Here's how the part is built. I have some questions about the finished solid (model axes, mm). Face numbers are marked on the shaded views. A direction names the side the tool comes from. Round coordinates to 2 decimals unless told otherwise and drop trailing zeros. Loops run counter-clockwise (first coordinate to the right, second up) from the corner with the lowest first, then second, coordinate; pieces in that order, holes last. Notation, with made-up numbers: M 23,18 L 46,18 A17 cw 46,51 Z; hole C -1.75,43.25 d4. An arc over 180 degrees is marked long. Answer as CSV lines item,"result".
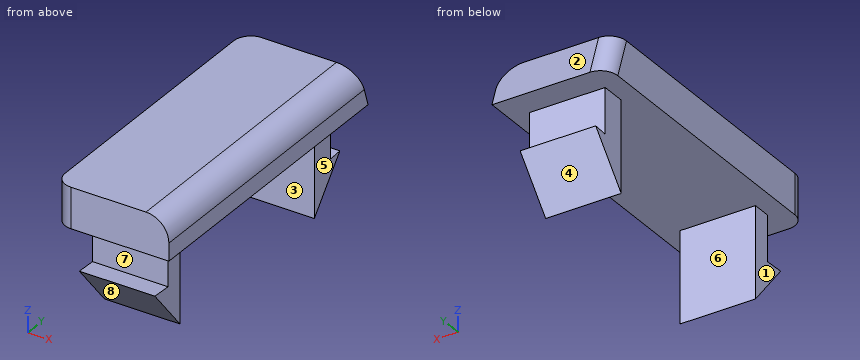
```python
from build123d import *

# Parameters (mm, degrees)
F1_DEPTH = 12.7
F2_DEPTH = 8.382
F3_R     = 3.679261
F4_R     = 5.08


with BuildPart() as f1:
    # F0 (on Right) → F1 (new body, symmetric)
    with BuildSketch(Plane.YZ):
        Polygon((30.308623, 31.392861), (-34.372479, 31.392861), (-34.724846, 31.392861), (-34.724846, 22.405792), (-28.332443, 22.405792), (-24.258062, 22.405792), (-20.550046, 22.405792), (-9.070974, 22.405792), (1.610943, 22.405792), (21.591455, 22.405792), (27.077377, 22.405792), (33.283076, 22.405792), align=None)
    extrude(amount=F1_DEPTH, both=True)

    # F0 (on Right) → F2 (join, symmetric)
    with BuildSketch(Plane.YZ):
        Polygon((30.308623, 31.392861), (-34.372479, 31.392861), (-34.724846, 31.392861), (-34.724846, 22.405792), (-28.332443, 22.405792), (-24.258062, 22.405792), (-20.550046, 22.405792), (-9.070974, 22.405792), (1.610943, 22.405792), (21.591455, 22.405792), (27.077377, 22.405792), (33.283076, 22.405792), align=None)
        Polygon((27.077377, 12.309055), (27.077377, 22.405792), (21.591455, 22.405792), (21.591455, 2.212318), (30.308623, 12.499893), align=None)
        Polygon((-24.258062, 22.405792), (-28.332443, 22.405792), (-28.332443, 12.309055), (-32.845773, 12.499893), (-24.258062, 2.212318), align=None)
    extrude(amount=F2_DEPTH, both=True)

    # F3
    f3_edges = [f1.edges().sort_by_distance(p)[0] for p in [
        (-12.7, -34.724846, 26.899327),
        (-12.7, 31.795849, 26.899327),
    ]]
    fillet(f3_edges, radius=F3_R)

    # F4
    f4_edges = [f1.edges().sort_by_distance(p)[0] for p in [
        (12.7, -2.208112, 31.392861),
    ]]
    fillet(f4_edges, radius=F4_R)


solid = f1.part
```
1. For P1, Ø8, axis at x = 0.5, z = 18, coming from the +Y side; P2, Ø2.5, axis at y = 24.5, z = 8, coming from the +X side; P3, Ø1, axis at x = -2, z = 20.5, coming from the -Y side, each with a flat end and sliding along its axis, tell me the tip position at first contact or that it passes through.
Evaluation:
P1,"stops at y = 27.08"
P2,"stops at x = 8.38"
P3,"stops at y = -28.33"
2. Which directions (+Z, -Z, +X, -X, +Y, -Y) give clear straight access to the entire face, cutting with the end or side of a thin tool? Please do the marked faces 1, 2, 3, 4 and 5.
Evaluation:
face 1,"-Z, -X, +Y, -Y"
face 2,"+Z, +X, -X, +Y"
face 3,"-Z, +X, -X"
face 4,"-Z, +X, -X, +Y"
face 5,"-Z, +X, +Y, -Y"
3. I want a section at D-D, the plane z = 9.5. Please give me the cut outline in (x, y).
Evaluation:
outline,"M -8.38,-30.34 L 8.38,-30.34 L 8.38,-24.26 L -8.38,-24.26 Z; M -8.38,21.59 L 8.38,21.59 L 8.38,27.77 L -8.38,27.77 Z"
4. If I drill on line 1 (Y direction, x = 3.5, z = 13); line 2 (Z direction, x = -11.25, y = 2); line 3 (Y direction, x = 7.5, z = 9.25), over which ranges is the centre line in solid material (lowest first)? Write a range as [from, to].
Evaluation:
line 1,"y = [-28.33, -24.26], [21.59, 27.08]"
line 2,"z = [22.41, 31.39]"
line 3,"y = [-30.13, -24.26], [21.59, 27.55]"
5. I want a section at C-C, the plane x = 3.5. Please give me the cut outline in (y, z).
Evaluation:
outline,"M -34.72,22.41 L -28.33,22.41 L -28.33,12.31 L -32.85,12.5 L -24.26,2.21 L -24.26,22.41 L 21.59,22.41 L 21.59,2.21 L 30.31,12.5 L 27.08,12.31 L 27.08,22.41 L 33.28,22.41 L 30.31,31.39 L -34.72,31.39 Z"
6. I want a section at A-A, the plane z = 18.5. Please give me the cut outline in (x, y).
Evaluation:
outline,"M -8.38,-28.33 L 8.38,-28.33 L 8.38,-24.26 L -8.38,-24.26 Z; M -8.38,21.59 L 8.38,21.59 L 8.38,27.08 L -8.38,27.08 Z"
7. We'd pull the mould along Z, two halves only. Please class the marked faces 6, 7 and 8: pulls with the +Z half, pulls with the -Z half, needs draft (parallel to the pull), parting line crosses it, or undercut.
Evaluation:
face 6,"needs draft"
face 7,"undercut"
face 8,"pulls with the -Z half"
8. I want a section at B-B, the plane y = -6.5. Please give me the cut outline in (x, z).
Evaluation:
outline,"M -12.7,22.41 L 12.7,22.41 L 12.7,26.31 A5.08 ccw 7.62,31.39 L -12.7,31.39 Z"
